Part model, mm, in its own coordinate system. A direction names the side the tool comes from. Round coordinates to 2 decimals unless told otherwise and drop trailing zeros. Loops run counter-clockwise (first coordinate to the right, second up) from the corner with the lowest first, then second, coordinate; pieces in that order, holes last. Notation, with made-up numbers: M 37.5,-21 L 87.5,-21 A18 ccw 87.5,2 Z; hole C 28.5,34 d1. An arc over 180 degrees is marked long. Put each result on its own line as item: value. Start each with the question number.
1) Slice it at D-D on x = -13. Give the cut face in (y, z).
2) Slice it at B-B on y = 2. Give the cut face in (x, z) (3 decimals).
3) Which spindle directions (+Z, -Z, +X, -X, +Y, -Y) get a long thin tool onto all of the face, cutting with end or side? Do faces 1 (the flat face through (18.788, 1.72, 32.396)), 2 (the flat face through (0, 0, 9)), 3 (the flat face through (0, 3, 10)). Say none if no direction does.
4) Slice it at C-C on y = -4.75. Give the cut face in (x, z), then the cut area to 3 significant figures.
5) Pull direction X, two halves, no side cores. Call faces 4 (the flat face through (-0.22, -1.37, 29.58)), 5 (the cylindrical face through (16.76, -0.97, 33.01)), 6 (the flat face through (-17.5, -2, 34)): +X half, -X half, draft (parallel to the pull), parting line (faces both ways), or undercut.
6) Probe line 1 along X through (y, z) = (0.75, 33); line 2 along Y through (x, z) = (-6, 14); line 3 along X through (y, z) = (2.5, 4.5). List the from-to ranges inside material, lowest first.
7) Slice it at A-A on z = 5. Give the cut face in (x, y), then the cut area to 3 significant figures.
8) Drop flat-ended pins along their axis: pin 1 Ø15 at (x, z) = (-9.5, 7.5) entering from -Y; pin 2 Ø1.5 at (x, z) = (0.5, 29.5) entering from -Y; pin 3 Ø2 at (y, z) = (-0.52, 34.07) entering from -X; pin 4 Ø21.5 at (x, z) = (9.5, 14) entering from +Y. Give the stop position or say it passes through.
Autodesk Inventor part; units mm, degrees
ref_plane "YZ Plane" through (0, 0, 0) normal (1, 0, 0) x (0, 1, 0)
ref_plane "XZ Plane" through (0, 0, 0) normal (0, 1, 0) x (-1, 0, 0)
ref_plane "XY Plane" through (0, 0, 0) normal (0, 0, 1) x (1, 0, 0)
sketch "スケッチ1" plane through (0, 0, 0) normal (0, 1, 0) x (-1, 0, 0)
  line L0 (21.5, 0) -> (-21.5, 0)
  line L1 (-21.5, 0) -> (-21.5, 25)
  line L2 (-21.5, 25) -> (21.5, 25)
  line L3 (21.5, 25) -> (21.5, 0)
  circle A0 centre (0, 5) radius 1.1
  circle A1 centre (13, 5) radius 1.1
  circle A2 centre (-13, 5) radius 1.1
  line L4 (0, 0) -> (0, 25) construction
  dimension "d0" = 43
  dimension "d1" = 13
  dimension "d2" = 2.2
  dimension "d3" = 5
  dimension "d6" = 25
extrude "押し出し1" add sketch "スケッチ1" along normal blind 3
sketch "スケッチ2" plane through (21.5, 0, 25) normal (1, 0, 0) x (0, 0, -1)
  line L0 (5.6249, 3) -> (6.4287, 0)
  line L1 (6.4287, 0) -> (-12.8898, -5.1764)
  line L2 (-12.8898, -5.1764) -> (-13.6936, -2.1764)
  line L3 (-13.6936, -2.1764) -> (5.6249, 3)
  line L4 (0, 3) -> (25, 3)
  line L5 (0, 0) -> (25, 0)
  line L6 (6.134, 1.1) -> (-6.5703, -2.3041) construction
  dimension "d7" = 20
extrude "押し出し2" add sketch "スケッチ2" against normal up to surface (43 mm away)
sketch "スケッチ3" plane through (21.5, 0, 0) normal (1, 0, 0) x (0, 0, -1)
  line L0 (-36.517, -6.8159) -> (-30.0178, -0.888)
  line L1 (-30.0178, -0.888) -> (-34.0611, 3.545)
  line L2 (-34.0611, 3.545) -> (-38.1247, -0.1614)
  line L3 (-38.1247, -0.1614) -> (-37.4508, -0.9002)
  line L4 (-37.4508, -0.9002) -> (-36.517, -6.8159)
  line L5 (-25, 3) -> (0, 3)
  line L6 (-25, 1.4928) -> (-25, 3)
  line L7 (-25, 1.4928) -> (-38.6936, -2.1764)
  line L8 (-38.6936, -2.1764) -> (-37.8898, -5.1764)
  line L9 (-37.8898, -5.1764) -> (-18.5713, 0)
  line L10 (-18.5713, 0) -> (0, 0)
  line L11 (0, 0) -> (0, 3)
  line L12 (-25, 1.4928) -> (-19.3751, 3)
  line L13 (-25, 1.4928) -> (-38.6936, -2.1764)
  point P0 (0, 0)
  point P1 (-31.5703, -2.3041)
  point P2 (-36.821, -4.89)
  point P3 (-37.308, -1.8051)
  point P4 (-33.4007, -3.9735)
  point P5 (-30.7774, -0.0552)
extrude "押し出し3" cut sketch "スケッチ3" against normal through all contours L9 L8 L7 L4 | L6 L5 L12
extrude "押し出し4" add sketch "スケッチ3" against normal up to surface (43 mm away) contours L4 L9 L0 | L4 L3 L2 L1 L7
sketch "スケッチ4" plane through (0, 0, 0) normal (1, 0, 0) x (0, 1, 0)
  line L0 (-0.9002, 37.4508) -> (-6.8159, 36.517)
  line L1 (-6.8159, 36.517) -> (-3.9735, 33.4007)
  line L2 (-3.9735, 33.4007) -> (0, 18.5713)
  line L3 (0, 18.5713) -> (0, 0)
  line L4 (0, 0) -> (3, 0)
  line L5 (3, 19.3751) -> (3, 0)
  line L6 (3, 19.3751) -> (-0.0552, 30.7774)
  line L7 (-0.0552, 30.7774) -> (3.545, 34.0611)
  line L8 (3.545, 34.0611) -> (-0.1614, 38.1247)
  line L9 (-0.1614, 38.1247) -> (-0.9002, 37.4508)
  line L10 (-0.0552, 30.7774) -> (-2.6391, 28.4206)
  point P0 (0, 0)
extrude "押し出し5" cut sketch "スケッチ4" along normal mid plane 24 contours L9 L8 L7 L10 L2 L1 L0
sketch "スケッチ6" plane through (12, 0, 0) normal (-1, 0, 0) x (0, 0, 1)
  line L0 (33.4007, -3.9735) -> (28.4206, -2.6391)
  line L1 (36.517, -6.8159) -> (33.4007, -3.9735)
  line L2 (37.4508, -0.9002) -> (36.517, -6.8159)
  line L3 (38.1247, -0.1614) -> (37.4508, -0.9002)
  line L4 (34.0611, 3.545) -> (38.1247, -0.1614)
  line L5 (30.7774, -0.0552) -> (34.0611, 3.545)
  line L6 (28.4206, -2.6391) -> (30.7774, -0.0552)
  point P0 (0, 0)
extrude "押し出し7" cut sketch "スケッチ6" against normal blind 4
sketch "スケッチ7" plane through (21.5, 0, 0) normal (1, 0, 0) x (0, 0, -1)
  circle A0 centre (-34.0712, -0.5247) radius 0.8 construction
  circle A1 centre (-34.0712, -0.5247) radius 1.15
  point P0 (0, 0)
  dimension "d21" = 2.3
extrude "押し出し8" cut sketch "スケッチ7" against normal up to surface (5.5 mm away)
sketch "スケッチ8" plane through (21.5, 0, 0) normal (1, 0, 0) x (0, 0, -1)
  circle A0 centre (-34.0712, -0.5247) radius 1.15
  circle A1 centre (-34.0712, -0.5247) radius 2
  point P0 (0, 0)
  dimension "d24" = 4
extrude "押し出し9" cut sketch "スケッチ8" against normal blind 4 contours A0 | A1
mirror "ミラー1" about plane through (0, 0, 0) normal (1, 0, 0) of "押し出し9", "押し出し8", "押し出し7"
properties part number "chest_cover_front"
Recorded:
1. outline: M -2.64,28.42 L 0,18.57 L 0,6.1 L 3,6.1 L 3,19.38 L 1.49,25 L -0.06,30.78 Z; M 0,0 L 3,0 L 3,3.9 L 0,3.9 Z
2. outline: M -21.5,0 L 21.5,0 L 21.5,23.107 L -21.5,23.107 Z; M -21.5,32.652 L -16,32.652 L -16,35.755 L -21.5,35.755 Z; M 16,32.652 L 21.5,32.652 L 21.5,35.755 L 16,35.755 Z; hole C -13,5 d2.2; hole C 0,5 d2.2; hole C 13,5 d2.2
3. face 1: +X, -X, +Y
3. face 2: -Z, +X, -X, -Y
3. face 3: -Z, +X, -X, +Y
4. outline: M -21.5,34.25 L -16,34.25 L -16,36.84 L -21.5,36.84 Z; M 16,34.25 L 21.5,34.25 L 21.5,36.84 L 16,36.84 Z
4. area: 28.5 mm2
5. face 4: undercut
5. face 5: draft
5. face 6: -X half
6. line 1: x = -17.5 to -16, 16 to 17.5
6. line 2: y = 0 to 3
6. line 3: x = -21.5 to -13.98, -12.02 to -0.98, 0.98 to 12.02, 13.98 to 21.5
7. outline: M -21.5,0 L -14.1,0 L -14.1,3 L -21.5,3 Z; M -11.9,0 L -1.1,0 L -1.1,3 L -11.9,3 Z; M 1.1,0 L 11.9,0 L 11.9,3 L 1.1,3 Z; M 14.1,0 L 21.5,0 L 21.5,3 L 14.1,3 Z
7. area: 109 mm2
8. pin 1: stops at y = 0
8. pin 2: stops at y = -2.28
8. pin 3: passes through
8. pin 4: stops at y = 3
